from build123d import *

# Parameters (mm, degrees)
EXTRUDE_1_DEPTH        = 175
PATTERN_LINEAR_1_COUNT = 3
PATTERN_LINEAR_1_PITCH = 160


with BuildPart() as part:
    # 草图1 → 凸台-拉伸1 (new, symmetric)
    with BuildSketch(Plane(origin=(0, 0, 0), x_dir=(0, 0, -1), z_dir=(1, 0, 0))):
        Polygon((0, -10), (0, 10), (7.2, 10), (7.2, 7.35), (2, 7.35), (2, -7.35), (7.2, -7.35), (7.2, -10), align=None)
    extrude(amount=EXTRUDE_1_DEPTH, both=True)

    # 草图5 → M3 开槽半沉头木螺钉的锥形沉头孔1 (revolve, cut)
    with BuildSketch(Plane(origin=(160, 0, -2), x_dir=(0, 1, 0), z_dir=(1, 0, 0))):
        Polygon((0, 0), (0, 2), (1.7, 2), (1.7, 1.6), (3.3, 0), align=None)
    hole_wizard_m3_1 = revolve(axis=Axis((160, 0, -8.35), (0, 0, 1)), mode=Mode.SUBTRACT)

    # 阵列(线性)1: M3 开槽半沉头木螺钉的锥形沉头孔1 ×3
    with Locations(*[(-i * PATTERN_LINEAR_1_PITCH, 0, 0) for i in range(1, PATTERN_LINEAR_1_COUNT)]):
        add(hole_wizard_m3_1, mode=Mode.SUBTRACT)


solid = part.part
Model file for the job. Use its own axes, mm. A direction names the side the tool comes from. Coordinates: 2 decimals unless noted, no trailing zeros. Write each loop counter-clockwise with the first axis right and the second up, starting at its lowest first coordinate (ties: lowest second). Pieces come first, ordered by that corner, then holes. Notation, with made-up numbers: (84, -40) - (119, -40) arc R30 ccw to (119, -11) - close; hole circle Ø11 at (86, -27.75). An arc over 180 degrees is marked (long way). Write each question's results on one line, items separated by ' | '. Start each with the question number.
1) Probe line 1 along X through (y, z) = (0, -0.2); line 2 along Y through (x, z) = (109, -4.5); line 3 along Y through (x, z) = (160, -0.3). List the from-to ranges inside material, lowest first. Write a range as from..to.
2) Flat gauge pins, fed straight in: P1, Ø7.5, axis at x = -24, y = -3.5, coming from the -Z side; P2, Ø5.5, axis at x = 0, y = 0, coming from the -Z side; P3, Ø3, axis at y = -4.5, z = -4, coming from the -X side. Where does each tip first touch, or does it go through?
3) Cut at A-A (x = -79.5). Write the cut outline in (y, z).
4) 3-axis set-ups, long thin cutter, end or side, ignore diameter. For faces 1 (the face through (2, 0, 0)), 2 (the face through (2, -3, -2)): which of +Z, -Z, +X, -X, +Y, -Y reach the whole face in a straight line?
Returned:
1) line 1: -175..-161.7, -158.3..-1.7, 1.7..158.3, 161.7..175 | line 2: -10..-7.35, 7.35..10 | line 3: -10..-1.7, 1.7..10
2) P1: z = -2 | P2: z = -1.45 | P3: through
3) outline: (-10, -7.2) - (-7.35, -7.2) - (-7.35, -2) - (7.35, -2) - (7.35, -7.2) - (10, -7.2) - (10, 0) - (-10, 0) - close
4) face 1: +Z, +X, -X, +Y, -Y | face 2: -Z, +X, -X
